The listing builds one solid part. Answer for the finished solid, in the listing's coordinates (mm). A direction names the side the tool comes from. Coordinates: 2 decimals unless noted, no trailing zeros. Order: outer loops, then holes, each group sorted by start corner. A loop starts at its lowest first (then second) coordinate and runs counter-clockwise, first axis right, second up. Notation, with made-up numbers: (33.25, 40) -> (59.25, 40) arc R19 ccw to (59.25, 46) -> close; hole circle Ø7 at (48, 75.5). An arc over 180 degrees is marked (long way). Return JSON: item names as keys, results as strings.
from build123d import *

# Parameters (mm, degrees)
SKETCH1_W           = 50.8
SKETCH1_H           = 31.75
BOSS_EXTRUDE1_DEPTH = 6.35
SKETCH2_R           = 9.525
SKETCH2_R_2         = 3.2385
BOSS_EXTRUDE2_DEPTH = 31.75
BOSS_EXTRUDE3_DEPTH = 31.75
SKETCH4_R           = 6.35
SKETCH4_R_2         = 3.2385
BOSS_EXTRUDE4_DEPTH = 12.7
CUT_EXTRUDE1_REACH  = 8.35
SKETCH5_R           = 2.54
SKETCH6_R           = 2.54
CUT_EXTRUDE2_DEPTH  = 35.925
SKETCH7_R           = 4.7625
CUT_EXTRUDE3_DEPTH  = 19.05


with BuildPart() as part:
    # Sketch1 → Boss-Extrude1 (new body)
    with BuildSketch(Plane(origin=(0, 0, 0), x_dir=(1, 0, 0), z_dir=(0, 1, 0))):
        with Locations((25.4, 15.875)):
            Rectangle(SKETCH1_W, SKETCH1_H)
    extrude(amount=BOSS_EXTRUDE1_DEPTH)



with BuildPart() as body_2:
    # Sketch2 → Boss-Extrude2 (new body)
    with BuildSketch(Plane.XY):
        with Locations((85.725, -19.05)):
            Circle(SKETCH2_R)
        with Locations((85.725, -19.05)):
            Circle(SKETCH2_R_2, mode=Mode.SUBTRACT)
    extrude(amount=-BOSS_EXTRUDE2_DEPTH)


with BuildPart() as part_1:
    add(part.part)

    add(body_2.part)  # Boss-Extrude3 merges body 2
    # Sketch3 → Boss-Extrude3 (add)
    with BuildSketch(Plane.XY):
        with BuildLine():
            Line((50.8, 3.175), (88.852564162, -10.05311346))
            ThreePointArc((88.852564162, -10.05311346), (76.82515217, -15.656132943), (82.067835176, -27.844928678))
            Line((82.067835176, -27.844928678), (15.104990042, 0))
            Line((15.104990042, 0), (15.104990042, 3.175))
            Line((15.104990042, 3.175), (50.8, 3.175))
        make_face()
    extrude(amount=-BOSS_EXTRUDE3_DEPTH)

    # Sketch4 → Boss-Extrude4 (add)
    with BuildSketch(Plane.XY):
        with Locations((85.725, -19.05)):
            Circle(SKETCH4_R)
        with Locations((85.725, -19.05)):
            Circle(SKETCH4_R_2, mode=Mode.SUBTRACT)
    extrude(amount=BOSS_EXTRUDE4_DEPTH)

    # Sketch5 → Cut-Extrude1 (cut, up to next)
    with BuildSketch(Plane.XZ, mode=Mode.PRIVATE) as cut_extrude1_sk1:
        with Locations((7.552495021, -7.9375)):
            Circle(SKETCH5_R)
    cut_extrude1_tool1 = extrude(cut_extrude1_sk1.sketch, amount=-CUT_EXTRUDE1_REACH, mode=Mode.PRIVATE) & part_1.part
    add(cut_extrude1_tool1.solids().sort_by_distance((7.552495, 0, -7.9375))[0], mode=Mode.SUBTRACT)
    # Sketch5 → Cut-Extrude1 (cut, up to next)
    with BuildSketch(Plane.XZ, mode=Mode.PRIVATE) as cut_extrude1_sk2:
        with Locations((7.552495021, -23.8125)):
            Circle(SKETCH5_R)
    cut_extrude1_tool2 = extrude(cut_extrude1_sk2.sketch, amount=-CUT_EXTRUDE1_REACH, mode=Mode.PRIVATE) & part_1.part
    add(cut_extrude1_tool2.solids().sort_by_distance((7.552495, 0, -23.8125))[0], mode=Mode.SUBTRACT)

    # Sketch6 → Cut-Extrude2 (cut, through all)
    with BuildSketch(Plane(origin=(0, 6.35, 0), x_dir=(1, 0, 0), z_dir=(0, 1, 0))):
        with Locations((43.247504979, 7.9375)):
            Circle(SKETCH6_R)
        with Locations((43.247504979, 23.8125)):
            Circle(SKETCH6_R)
    extrude(amount=-CUT_EXTRUDE2_DEPTH, mode=Mode.SUBTRACT)

    # Sketch7 → Cut-Extrude3 (cut)
    with BuildSketch(Plane(origin=(0, -19.05, 0), x_dir=(1, 0, 0), z_dir=(0, 1, 0))):
        with Locations((43.247504979, 23.8125)):
            Circle(SKETCH7_R)
        with Locations((43.247504979, 7.9375)):
            Circle(SKETCH7_R)
    extrude(amount=CUT_EXTRUDE3_DEPTH, mode=Mode.SUBTRACT)


solid = part_1.part
1. The part is cut by section C-C on x = 26.5. Give the vertices of the cut face in (y, z).
Answer block:
{"outline": "(-4.74, -31.75) -> (6.35, -31.75) -> (6.35, 0) -> (-4.74, 0) -> close"}
2. Each of these flat-tipped pins is pushed along its axis until it touches: pin 1 Ø5 at (y, z) = (-23.5, -12) entering from -X; pin 2 Ø7.5 at (x, z) = (43.5, -22.5) entering from -Y; pin 3 Ø12 at (x, z) = (49, -6) entering from -Y. Where does it stop, or does it pass through?
Answer block:
{"pin 1": "stops at x = 65.61", "pin 2": "stops at y = -13.13", "pin 3": "stops at y = -16.59"}
3. For faces 4 (the face through (91.59, -21.48, 6.26)), 5 (the face through (49.06, -14.12, -15.65)), 6 (the face through (50.8, 5, -16)), 7 (the face through (47.79, -5.42, -9.37)), determine the directions among +Z, -Z, +X, -X, +Y, -Y from which every point of the face is accessible in a straight line to the end or side of a thin tool.
Answer block:
{"face 4": "+Z", "face 5": "+Z, -Z, -X, -Y", "face 6": "+Z, -Z, +X, +Y", "face 7": "-Y"}
4. The part is cut by section A-A on y = -21. Give the vertices of the cut face in (x, z), and give its area (3 significant figures).
Answer block:
{"outline": "(65.61, -31.75) -> (83.14, -31.75) -> (83.14, 12.7) -> (79.68, 12.7) -> (79.68, 0) -> (65.61, 0) -> close; (88.31, -31.75) -> (95.05, -31.75) -> (95.05, 0) -> (91.77, 0) -> (91.77, 12.7) -> (88.31, 12.7) -> close", "area": "858 mm2"}
5. Consider line 1 (Z direction, x = 62.5, y = -8.5); line 2 (X direction, y = -20.5, z = -14.5); line 3 (X direction, y = 4, z = -17). Determine where each line is inside the solid, lowest interval first. Write a range as from..to.
Answer block:
{"line 1": "z = -31.75..0", "line 2": "x = 64.4..82.83, 88.62..95.14", "line 3": "x = 0..50.8"}
6. Determine the mould class of faces 1 (the face through (47.647, -5.417, -21.988)), 2 (the face through (94.547, -22.642, -15.653)), 3 (the face through (25, 6.35, -16)) for opening direction X: pulls with the +X half, pulls with the -X half, needs draft (parallel to the pull), parting line crosses it, or undercut.
Answer block:
{"face 1": "undercut", "face 2": "parting line crosses it", "face 3": "needs draft"}
